from build123d import *

# Parameters (mm, degrees)
SALIENTE_EXTRUIR1_DEPTH = 25.4
CROQUIS2_W              = 101.6
CROQUIS2_H              = 25.4
SALIENTE_EXTRUIR2_DEPTH = 101.6
CROQUIS3_R              = 50.8
SALIENTE_EXTRUIR3_DEPTH = 25.4
CROQUIS4_R              = 38.1
CORTAR_EXTRUIR1_DEPTH   = 204.2
CROQUIS5_W              = 25.4
CROQUIS5_H              = 101.6
SALIENTE_EXTRUIR4_DEPTH = 101.6
CROQUIS6_R              = 50.8
SALIENTE_EXTRUIR5_DEPTH = 25.4
CROQUIS7_R              = 38.1
CORTAR_EXTRUIR3_DEPTH   = 26.4


with BuildPart() as part:
    # Croquis1 → Saliente-Extruir1 (new body)
    with BuildSketch(Plane(origin=(0, 0, 0), x_dir=(1, 0, 0), z_dir=(0, 1, 0))):
        with BuildLine():
            Line((0, 0), (0, 101.6))
            Line((0, 101.6), (158.496, 101.6))
            ThreePointArc((158.496, 101.6), (261.948550515, 58.748550515), (304.8, -44.704))
            Line((304.8, -44.704), (304.8, -101.6))
            Line((304.8, -101.6), (203.2, -101.6))
            Line((203.2, -101.6), (203.2, -32.004))
            ThreePointArc((203.2, -32.004), (193.826245425, -9.373754575), (171.196, 0))
            Line((171.196, 0), (0, 0))
        make_face()
    extrude(amount=SALIENTE_EXTRUIR1_DEPTH)

    # Croquis2 → Saliente-Extruir2 (add)
    with BuildSketch(Plane.XZ):
        with Locations((254, 88.9)):
            Rectangle(CROQUIS2_W, CROQUIS2_H)
    extrude(amount=SALIENTE_EXTRUIR2_DEPTH)

    # Croquis3 → Saliente-Extruir3 (add)
    with BuildSketch(Plane.XY.offset(101.6)):
        with Locations((254, -101.6)):
            Circle(CROQUIS3_R)
    extrude(amount=-SALIENTE_EXTRUIR3_DEPTH)

    # Croquis4 → Cortar-Extruir1 (cut, through all)
    with BuildSketch(Plane.XY.offset(101.6)):
        with Locations((254, -101.6)):
            Circle(CROQUIS4_R)
    extrude(amount=-CORTAR_EXTRUIR1_DEPTH, mode=Mode.SUBTRACT)

    # Croquis5 → Saliente-Extruir4 (add)
    with BuildSketch(Plane(origin=(0, 25.4, 0), x_dir=(1, 0, 0), z_dir=(0, 1, 0))):
        with Locations((12.7, 50.8)):
            Rectangle(CROQUIS5_W, CROQUIS5_H)
    extrude(amount=SALIENTE_EXTRUIR4_DEPTH)

    # Croquis6 → Saliente-Extruir5 (add)
    with BuildSketch(Plane(origin=(25.4, 0, 0), x_dir=(0, 0, -1), z_dir=(1, 0, 0))):
        with Locations((50.8, 127)):
            Circle(CROQUIS6_R)
    extrude(amount=-SALIENTE_EXTRUIR5_DEPTH)

    # Croquis7 → Cortar-Extruir3 (cut, through all)
    with BuildSketch(Plane(origin=(25.4, 0, 0), x_dir=(0, 0, -1), z_dir=(1, 0, 0))):
        with Locations((50.8, 127)):
            Circle(CROQUIS7_R)
    extrude(amount=-CORTAR_EXTRUIR3_DEPTH, mode=Mode.SUBTRACT)


solid = part.part
CAD build for the part. Positions are in the model's coordinates, mm. A direction names the side the tool comes from. Coordinates: 2 decimals unless noted, no trailing zeros. Loops run counter-clockwise (first coordinate to the right, second up) from the corner with the lowest first, then second, coordinate; pieces in that order, holes last. Notation, with made-up numbers: (-5, 88.25) - (17, 88.25) arc R19 cw to (17, 110.25) - close; hole circle Ø9 at (52.5, 59.5). An arc over 180 degrees is marked (long way). Use one line per item in the form item = value. Start each with the question number.
1) Tool access for faces 4 (the face through (203.2, -23, 82)), 5 (the face through (167, 25.4, -24)), 6 (the face through (253, -58, 76.2)): list every direction of +Z, -Z, +X, -X, +Y, -Y with a clear straight run to the whole face (end or side of a thin tool).
2) Band-saw the part on A-A (z = -50.8). Give the cut face in (x, y).
3) Drill centre lines: L1, parallel to Y at x = 254, z = 83.5; L2, parallel to Y at x = 157, z = -65.5. Where is each one in solid material? Low to high. Write a range as from..to.
4) Band-saw the part on C-C (y = -37). Give the cut face in (x, z), and give its area (3 significant figures).
5) Band-saw the part on B-B (x = 286.5). Give the cut face in (y, z).
6) Flat gauge pins, fed straight in: pin 1 (6 mm diameter, centred on x = 160.5, z = -47, fed in from -Y); pin 2 (2 mm diameter, centred on x = 227, y = 19.5, fed in from -Z); pin 3 (6 mm diameter, centred on x = 200.5, z = 30.5, fed in from +Y). Where does each tip first touch, or does it go through?
7) Two-plate mould, pull along Y, no slides. Class faces 1 (the face through (12.878, 89.806, -42.541)), 2 (the face through (253, -42, 101.6)), 3 (the face through (155, 0, -34)): +Y half, -Y half, draft (parallel to the pull), parting line (faces both ways), or undercut.
8) Band-saw the part on D-D (x = 32.5). Give the cut face in (y, z).
Check values:
q1.face_4 = +Z, -X, +Y, -Y
q1.face_5 = +Z, -Z, +X, +Y
q1.face_6 = -Z, +X, -X, -Y
q2.outline = (0, 0) - (269.33, 0) - (269.33, 25.4) - (25.4, 25.4) - (25.4, 88.9) - (0, 88.9) - close; (0, 165.1) - (25.4, 165.1) - (25.4, 177.8) - (0, 177.8) - close
q3.L1 = -152.4..-139.7, -63.5..25.4
q3.L2 = 0..25.4
q4.outline = (203.2, 76.2) - (304.8, 76.2) - (304.8, 101.6) - (203.2, 101.6) - close
q4.area = 2,580 mm2
q5.outline = (-140.64, 76.2) - (-121.48, 76.2) - (-121.48, 101.6) - (-140.64, 101.6) - close; (-81.72, 76.2) - (0, 76.2) - (0, -26.15) - (25.4, -26.15) - (25.4, 101.6) - (-81.72, 101.6) - close
q6.pin_1 = 0
q6.pin_2 = -85.1
q6.pin_3 = 25.4
q7.face_1 = undercut
q7.face_2 = draft
q7.face_3 = -Y half
q8.outline = (0, -101.6) - (25.4, -101.6) - (25.4, 0) - (0, 0) - close
